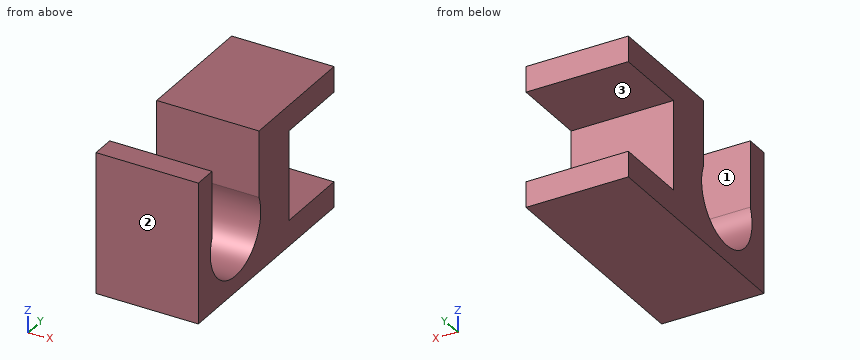
```python
from build123d import *

# Parameters (mm, degrees)
F0_W     = 25.4
F0_H     = 31.75
F2_DEPTH = 6.35
F1_W     = 25.4
F1_H     = 12.7
F3_DEPTH = 28.575
F4_W     = 25.4
F4_H     = 31.75
F5_DEPTH = 6.35
F6_W     = 25.4
F6_H     = 34.925
F7_DEPTH = 25.4
F8_W     = 19.7909511626
F8_H     = 16.4385318786
F9_DEPTH = 33.782


with BuildPart() as f2:
    # F0 (on Top) → F2 (new body)
    with BuildSketch(Plane.XY):
        with Locations((-12.7, -7.5953084708)):
            Rectangle(F0_W, F0_H)
    extrude(amount=F2_DEPTH)

    # F1 (on face) → F3 (join)
    with BuildSketch(Plane.XY):
        with Locations((-12.7, -17.1203084708)):
            Rectangle(F1_W, F1_H)
    extrude(amount=F3_DEPTH)

    # F4 (on face) → F5 (join)
    with BuildSketch(Plane.XY.offset(28.575)):
        with Locations((-12.7, -7.5953084708)):
            Rectangle(F4_W, F4_H)
    extrude(amount=F5_DEPTH)

    # F6 (on Right) → F7 (join)
    with BuildSketch(Plane.YZ):
        with Locations((-36.1703084708, 17.4625)):
            Rectangle(F6_W, F6_H)
    extrude(amount=-F7_DEPTH)

    # F8 (on face) → F9 (cut)
    with BuildSketch(Plane.YZ):
        with Locations((-33.2048367709, 26.7057340607)):
            Rectangle(F8_W, F8_H)
        with BuildLine():
            Line((-23.3093611896, 18.4864681214), (-43.1003123522, 18.4864681214))
            ThreePointArc((-43.1003123522, 18.4864681214), (-33.2048367709, 4.0030932476), (-23.3093611896, 18.4864681214))
        make_face()
    extrude(amount=-F9_DEPTH, mode=Mode.SUBTRACT)


solid = f2.part
```
Check sheet for the modelled part. Datum: model origin and axes. Units: mm. Face numbers are marked on the shaded views. A direction names the side the tool comes from. Give positions to 0.01 mm unless a question says otherwise; leave off trailing zeros. Order: outer loops, then holes, each group sorted by start corner. A loop starts at its lowest first (then second) coordinate and runs counter-clockwise, first axis right, second up. Notation, with made-up numbers: M -13,41.25 L 13,41.25 A24 cw 13,77.25 Z; hole C 41,84 d9. An arc over 180 degrees is marked long. Answer in a Markdown table with one row per item.
1) Cross-section at A-A, the plane z = 29.5. Enter the section's corners in (x, y), plus the area to 3 significant figures.
Filled sheet:
| item | result |
|---|---|
| outline | M -25.4,-48.87 L 0,-48.87 L 0,-43.1 L -25.4,-43.1 Z; M -25.4,-23.31 L 0,-23.31 L 0,8.28 L -25.4,8.28 Z |
| area | 949 mm2 |
2) Cross-section at D-D, the plane y = -24. Enter the section's corners in (x, z), plus the area to 3 significant figures.
Filled sheet:
| item | result |
|---|---|
| outline | M -25.4,0 L 0,0 L 0,9.32 L -25.4,9.32 Z |
| area | 237 mm2 |
3) Thickness scan on L1, parallel to Z at x = -19, y = -5 (3 decimals); L2, parallel to Y at x = -1.25, z = 25; L3, parallel to Y at x = -19, z = 33.5. Record the ranges inside material, lowest first. Write a range as [from, to].
Filled sheet:
| item | result |
|---|---|
| L1 | z = [0, 6.35], [28.575, 34.925] |
| L2 | y = [-48.87, -43.1], [-23.31, -10.77] |
| L3 | y = [-48.87, -43.1], [-23.31, 8.28] |
4) Cross-section at B-B, the plane y = 2.5. Enter the section's corners in (x, z) (3 decimals).
Filled sheet:
| item | result |
|---|---|
| outline | M -25.4,0 L 0,0 L 0,6.35 L -25.4,6.35 Z; M -25.4,28.575 L 0,28.575 L 0,34.925 L -25.4,34.925 Z |
5) Access from +Z, -Z, +X, -X, +Y, -Y to the whole of each face (thin tool, end or side, straight path). Record for the marked faces 1, 2 and 3.
Filled sheet:
| item | result |
|---|---|
| face 1 | +Z, +X, -X |
| face 2 | +Z, -Z, +X, -X, -Y |
| face 3 | +X, -X, +Y |
6) Gauge pin test, flat ends, axial feed: P1, Ø10, axis at x = -18, z = 12.5, coming from the +Y side; P2, Ø2, axis at x = -18.5, y = -40.5, coming from the +Z side; P3, Ø19, axis at y = -33.2, z = 14.63, coming from the +X side (3 decimals). Record the tip position at first contact, or that the pin passes through.
Filled sheet:
| item | result |
|---|---|
| P1 | stops at y = -10.77 |
| P2 | stops at z = 7.99 |
| P3 | passes through |
7) Cross-section at C-C, the plane x = -11.5. Enter the section's corners in (y, z) (3 decimals).
Filled sheet:
| item | result |
|---|---|
| outline | M -48.87,0 L 8.28,0 L 8.28,6.35 L -10.77,6.35 L -10.77,28.575 L 8.28,28.575 L 8.28,34.925 L -23.309,34.925 L -23.309,18.486 A10.622 cw long -43.1,18.486 L -43.1,34.925 L -48.87,34.925 Z |
